```python
from build123d import *

# Parameters (mm, degrees)
SKETCH1_W           = 20
SKETCH1_H           = 250
BOSS_EXTRUDE1_DEPTH = 20
BOSS_EXTRUDE2_DEPTH = 20
BOSS_EXTRUDE3_DEPTH = 20
BOSS_EXTRUDE4_DEPTH = 20


with BuildPart() as part:
    # Sketch1 → Boss-Extrude1 (new body)
    with BuildSketch(Plane.XY):
        Rectangle(SKETCH1_W, SKETCH1_H)
    extrude(amount=BOSS_EXTRUDE1_DEPTH)

    # Sketch2 → Boss-Extrude2 (add)
    with BuildSketch(Plane.XY.offset(20)):
        Polygon((10, -125), (10, -105), (30, -125), align=None)
    boss_extrude2 = extrude(amount=-BOSS_EXTRUDE2_DEPTH)

    # Mirror2: Boss-Extrude2 across plane
    add(boss_extrude2.mirror(Plane(origin=(0, 0, 0), x_dir=(0, 0, 1), z_dir=(1, 0, 0))))

    # Sketch3 → Boss-Extrude3 (add)
    with BuildSketch(Plane(origin=(10, 0, 0), x_dir=(0, 0, -1), z_dir=(1, 0, 0))):
        Polygon((-20, -105), (-20, -125), (-40, -125), align=None)
    boss_extrude3 = extrude(amount=-BOSS_EXTRUDE3_DEPTH)

    # Mirror3: Boss-Extrude3 across plane
    add(boss_extrude3.mirror(Plane(origin=(0, 0, 10), x_dir=(1, 0, 0), z_dir=(0, 0, -1))))

    # Sketch4 → Boss-Extrude4 (add)
    with BuildSketch(Plane.XY.offset(20)):
        Polygon((-10, 125), (-20, 125), (-10, 65), align=None)
    boss_extrude4 = extrude(amount=-BOSS_EXTRUDE4_DEPTH)

    # Mirror4: Boss-Extrude4 across plane
    add(boss_extrude4.mirror(Plane(origin=(0, 0, 0), x_dir=(0, 0, 1), z_dir=(1, 0, 0))))


solid = part.part
```
CAD build for the part. Positions are in the model's coordinates, mm. A direction names the side the tool comes from. Coordinates: 2 decimals unless noted, no trailing zeros. Loops run counter-clockwise (first coordinate to the right, second up) from the corner with the lowest first, then second, coordinate; pieces in that order, holes last. Notation, with made-up numbers: (60, 32.5) - (109, 32.5) arc R25 ccw to (109, 64.5) - close; hole circle Ø4 at (-21.5, 6.5). An arc over 180 degrees is marked (long way). Use CSV: the item, a comma, the result in double quotes. Start each with the question number.
Q1. Cut at C-C, the plane z = -4.5. List the corners of the cut face in (x, y), then the cut area to 3 significant figures.
Q2. Cut at B-B, the plane y = -18. List the corners of the cut face in (x, z), then the cut area to 3 significant figures.
Q3. 3-axis set-ups, long thin cutter, end or side, ignore diameter. For faces 1 (the flat face through (-10, -119, -5)), 2 (the flat face through (20, -115, 10)), 3 (the flat face through (15, -119, 0)), 4 (the flat face through (-10, -21, 10)): which of +Z, -Z, +X, -X, +Y, -Y reach the whole face in a straight line?
Q4. Drop flat-ended pins along their axis: P1, Ø5, axis at x = 12, y = -98, coming from the -Z side; P2, Ø6, axis at y = -34, z = 9.5, coming from the +X side; P3, Ø1.5, axis at x = -2.5, z = 21.5, coming from the +Y side. Give the stop position or say it passes through.
Q5. Probe probe 1 along Z at (x, y) = (11, -111); probe 2 along X at (y, z) = (-55.5, 1); probe 3 along Y at (x, z) = (-2.5, 27). List the from-to ranges inside material, lowest first. Write a range as from..to.
Q6. Cut at A-A, the plane x = -12.5. List the corners of the cut face in (y, z), then the cut area to 3 significant figures.
Q7. Two-plate mould, pull along Y, no slides. Class faces 5 (the flat face through (-16, -119, 0)), 6 (the flat face through (0, -115, 30)), 7 (the flat face through (10, -21, 10)): +Y half, -Y half, draft (parallel to the pull), parting line (faces both ways), or undercut.
Q8. Cut at D-D, the plane x = 7. List the corners of the cut face in (y, z).
Here are the results:
1,outline,"(-10, -125) - (10, -125) - (10, -109.5) - (-10, -109.5) - close"
1,area,"310 mm2"
2,outline,"(-10, 0) - (10, 0) - (10, 20) - (-10, 20) - close"
2,area,"400 mm2"
3,face 1,"-Z, -X, +Y, -Y"
3,face 2,"+Z, -Z, +X"
3,face 3,"-Z, +X, +Y, -Y"
3,face 4,"+Z, -Z, -X"
4,P1,"z = 0"
4,P2,"x = 10"
4,P3,"y = -105.75"
5,probe 1,"0..20"
5,probe 2,"-10..10"
5,probe 3,"-125..-112"
6,outline,"(-125, 0) - (-107.5, 0) - (-107.5, 20) - (-125, 20) - close; (80, 0) - (125, 0) - (125, 20) - (80, 20) - close"
6,area,"1,250 mm2"
7,face 5,"draft"
7,face 6,"+Y half"
7,face 7,"undercut"
8,outline,"(-125, -20) - (-105, 0) - (125, 0) - (125, 20) - (-105, 20) - (-125, 40) - close"
